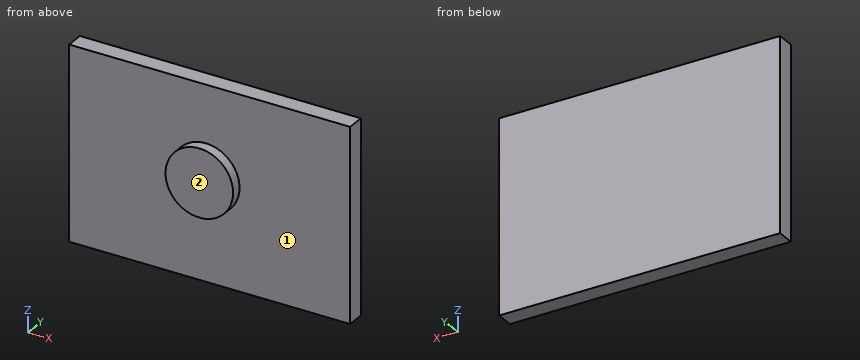
```python
from build123d import *

# Parameters (mm, degrees)
F0_W     = 79.294
F0_H     = 54.2539670305
F1_DEPTH = 5
F2_R     = 9.5370045267
F3_DEPTH = 3


# Not quite as in the source:
# - the program builds the solid bodies; features that only make, move or delete a surface that nothing else refers to are left out


with BuildPart() as f1:
    # F0 (on Front) → F1 (new body)
    with BuildSketch(Plane.XZ):
        with Locations((1.0885317774, -1.4516480646)):
            Rectangle(F0_W, F0_H)
    extrude(amount=-F1_DEPTH)

    # F2 (on face) → F3 (join)
    with BuildSketch(Plane.XZ):
        Circle(F2_R)
    extrude(amount=F3_DEPTH)


solid = f1.part
```
Geometry: final body of the model. Coordinates: model frame, mm. Face numbers are marked on the shaded views. A direction names the side the tool comes from. Round coordinates to 2 decimals unless told otherwise and drop trailing zeros. Loops run counter-clockwise (first coordinate to the right, second up) from the corner with the lowest first, then second, coordinate; pieces in that order, holes last. Notation, with made-up numbers: (-21.75, 59) -> (24.25, 59) arc R18 ccw to (24.25, 90) -> close; hole circle Ø9 at (-35, 30.25). An arc over 180 degrees is marked (long way). Write each question's results on one line, items separated by ' | '.
Item 1: Line query: probe 1 along Y at (x, z) = (33, -21); probe 2 along X at (y, z) = (-2.25, 6). Output: solid intervals per line, ascending. Write a range as [from, to].
Answers below:
probe 1: y = [0, 5] | probe 2: x = [-7.41, 7.41]
Item 2: Pin query (flat end, axial travel): pin 1 Ø1.5 at (x, z) = (26.5, 8) entering from -Y; pin 2 Ø1 at (x, y) = (-3, -1.5) entering from -Z. Return the tip coordinate at first contact, or that it passes through.
Answers below:
pin 1: stops at y = 0 | pin 2: stops at z = -9.2
Item 3: Cut plane D-D on x = -12. Return the cut outline in (y, z).
Answers below:
outline: (0, -28.58) -> (5, -28.58) -> (5, 25.68) -> (0, 25.68) -> close
Item 4: Cut plane B-B on z = 0. Return the cut outline in (x, y), and give its area (3 significant figures).
Answers below:
outline: (-38.56, 0) -> (-9.54, 0) -> (-9.54, -3) -> (9.54, -3) -> (9.54, 0) -> (40.74, 0) -> (40.74, 5) -> (-38.56, 5) -> close | area: 454 mm²
Item 5: Set-up query: the marked faces 1 and 2. Return all of +Z, -Z, +X, -X, +Y, -Y with unobstructed straight access to the full face (end or side cutting, diameter ignored); none if empty.
Answers below:
face 1: -Y | face 2: +Z, -Z, +X, -X, -Y
Item 6: Cut plane A-A on x = 0. Return the cut outline in (y, z).
Answers below:
outline: (-3, -9.54) -> (0, -9.54) -> (0, -28.58) -> (5, -28.58) -> (5, 25.68) -> (0, 25.68) -> (0, 9.54) -> (-3, 9.54) -> close
Item 7: Cut plane C-C on y = -1.5. Return the cut outline in (x, z).
Answers below:
outline: circle Ø19.07 at (0, 0)
